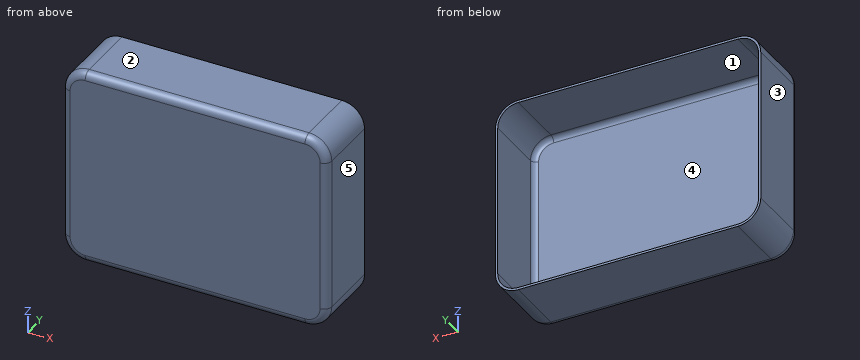
from build123d import *

# Parameters (mm, degrees)
SKETCH_1_W      = 350
SKETCH_1_H      = 260
EXTRUDE_1_DEPTH = 90
FILLET_1_R      = 30
FILLET_2_R      = 10
SHELL_1_T       = -3


with BuildPart() as part:
    # 草圖1 → 填料-伸長1 (new body)
    with BuildSketch(Plane(origin=(0, 0, 0), x_dir=(1, 0, 0), z_dir=(0, 1, 0))):
        Rectangle(SKETCH_1_W, SKETCH_1_H)
    extrude(amount=EXTRUDE_1_DEPTH)

    # 圓角1
    fillet_1_edges = [part.edges().sort_by_distance(p)[0] for p in [
        (175, 45, 130),
        (-175, 45, 130),
        (-175, 45, -130),
        (175, 45, -130),
    ]]
    fillet(fillet_1_edges, radius=FILLET_1_R)

    # 圓角2
    fillet_2_edges = [part.edges().sort_by_distance(p)[0] for p in [
        (-175, 0, 0),
        (175, 0, 0),
        (0, 0, 130),
        (0, 0, -130),
        (166.213203436, 0, 121.213203436),
        (166.213203436, 0, -121.213203436),
        (-166.213203436, 0, 121.213203436),
        (-166.213203436, 0, -121.213203436),
    ]]
    fillet(fillet_2_edges, radius=FILLET_2_R)

    # 薄殼1
    shell_1_openings = [part.faces().sort_by_distance(p)[0] for p in [
        (0, 90, 0),
    ]]
    offset(amount=SHELL_1_T, openings=shell_1_openings, kind=Kind.INTERSECTION)


solid = part.part
Source: CAD feature listing. Evaluate the final solid. Frame: model axes, mm. Face numbers are marked on the shaded views. A direction names the side the tool comes from. Round coordinates to 2 decimals unless told otherwise and drop trailing zeros. Loops run counter-clockwise (first coordinate to the right, second up) from the corner with the lowest first, then second, coordinate; pieces in that order, holes last. Notation, with made-up numbers: (3, 65.25) -> (41, 65.25) arc R23 cw to (41, 87.25) -> close; hole circle Ø4 at (-27.75, 86). An arc over 180 degrees is marked (long way). Answer as a JSON object with one key per item and string values. Group by question number.
Q1. Ray query, line 1 (Z direction, x = 0.5, y = 56); line 2 (X direction, y = 39.5, z = 32.5); line 3 (Y direction, x = 81.5, z = -57). Return the intervals inside material, ascending. Write a range as from..to.
Q2. Section query B-B (x = -98). Output: boundary loops of the cut face in (y, z).
Q3. Section query C-C (z = 75). Output: boundary loops of the cut face in (x, y).
Q4. Access query for the marked faces 4 and 5. Directions: +Z, -Z, +X, -X, +Y, -Y. A direction counts if a zero-diameter tool reaches every point of the face in a straight line with its end or side. Return the directions, or none.
Q5. Section query A-A (y = 27). Output: boundary loops of the cut face in (x, z), plus the area to 3 significant figures.
Q6. Mould query, pull axis Z, two halves, no side actions, for the marked faces 1, 2 and 3. Classes: pulls with the +Z half, pulls with the -Z half, needs draft (parallel to the pull), parting line crosses it, or undercut.
Completed:
{
 "1": {"line 1": "-130..-127, 127..130", "line 2": "-175..-172, 172..175", "line 3": "0..3"},
 "2": {"outline": "(0, -120) arc R10 ccw to (10, -130) -> (90, -130) -> (90, -127) -> (10, -127) arc R7 cw to (3, -120) -> (3, 120) arc R7 cw to (10, 127) -> (90, 127) -> (90, 130) -> (10, 130) arc R10 ccw to (0, 120) -> close"},
 "3": {"outline": "(-175, 10) arc R10 ccw to (-165, 0) -> (165, 0) arc R10 ccw to (175, 10) -> (175, 90) -> (172, 90) -> (172, 10) arc R7 cw to (165, 3) -> (-165, 3) arc R7 cw to (-172, 10) -> (-172, 90) -> (-175, 90) -> close"},
 "4": {"face 4": "+Y", "face 5": "+Z, -Z, +X, +Y, -Y"},
 "5": {"outline": "(-175, -100) arc R30 ccw to (-145, -130) -> (145, -130) arc R30 ccw to (175, -100) -> (175, 100) arc R30 ccw to (145, 130) -> (-145, 130) arc R30 ccw to (-175, 100) -> close; hole (-172, -100) arc R27 ccw to (-145, -127) -> (145, -127) arc R27 ccw to (172, -100) -> (172, 100) arc R27 ccw to (145, 127) -> (-145, 127) arc R27 ccw to (-172, 100) -> close", "area": "3,480 mm²"},
 "6": {"face 1": "undercut", "face 2": "pulls with the +Z half", "face 3": "needs draft"}
}
